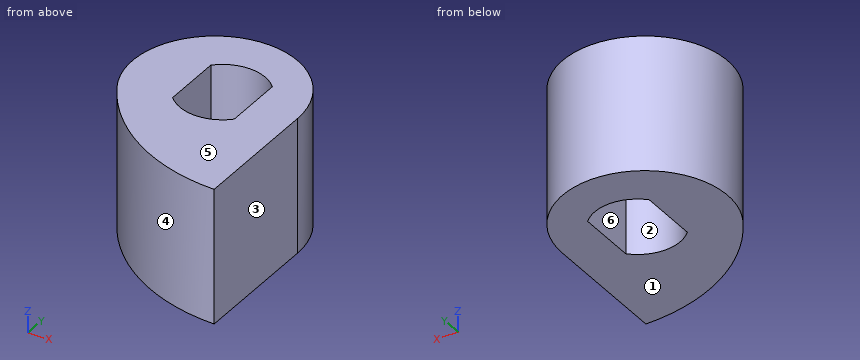
from build123d import *

# Parameters (mm, degrees)
EXTRUDE_935_DEPTH      = 4.5
EXTRUDE_935_DEPTH_BACK = 4.5


with BuildPart() as part:
    # Эскиз1 → Extrude 935 (new, two sides: drawn at the far end of the back side and taken through both)
    with BuildSketch(Plane.XY.offset(-EXTRUDE_935_DEPTH_BACK)):
        with BuildLine():
            Line((5, 0), (5, -8.660254038))
            ThreePointArc((5, -8.660254038), (-0.911767719, -7.082761379), (-5.251705953, -2.769709468))
            ThreePointArc((-5.251705953, -2.769709468), (-1.934506406, 5.309631943), (5, 0))
        make_face()
        with BuildLine():
            Line((-2.05, 1.979898987), (-2.05, -1.979898987))
            ThreePointArc((-2.05, -1.979898987), (0, -2.85), (2.05, -1.979898987))
            Line((2.05, -1.979898987), (2.05, 1.979898987))
            ThreePointArc((2.05, 1.979898987), (0, 2.85), (-2.05, 1.979898987))
        make_face(mode=Mode.SUBTRACT)
    extrude(amount=EXTRUDE_935_DEPTH + EXTRUDE_935_DEPTH_BACK)


solid = part.part
Model file for the job. Use its own axes, mm. Face numbers are marked on the shaded views. A direction names the side the tool comes from. Give positions to 0.01 mm unless a question says otherwise; leave off trailing zeros. Loops run counter-clockwise (first coordinate to the right, second up) from the corner with the lowest first, then second, coordinate; pieces in that order, holes last.
Item 1: Drop a flat-ended pin along its axis: P1, Ø2, axis at x = -4.5, z = -0.5, coming from the -Y side. Give the stop position or say it passes through.
Check values:
P1: stops at y = -5.07
Item 2: Slice it at C-C (x = -0.5). Write the cut outline in (y, z).
Check values:
outline: (-7.31, -4.5) - (-2.81, -4.5) - (-2.81, 4.5) - (-7.31, 4.5) - close; (2.81, -4.5) - (5.5, -4.5) - (5.5, 4.5) - (2.81, 4.5) - close
Item 3: Mould opens along X. For the marked faces 3, 4, 5 and 6 say: +X half, -X half, draft (parallel to the pull), parting line (faces both ways), or undercut.
Check values:
face 3: +X half
face 4: -X half
face 5: draft
face 6: undercut
Item 4: Slice it at B-B (y = 0.75). Write the cut outline in (x, z).
Check values:
outline: (-5.95, -4.5) - (-2.05, -4.5) - (-2.05, 4.5) - (-5.95, 4.5) - close; (2.05, -4.5) - (4.95, -4.5) - (4.95, 4.5) - (2.05, 4.5) - close
Item 5: Drill centre lines: line 1 along X through (y, z) = (1.5, 0.75); line 2 along Y through (x, z) = (-0.5, -3.75); line 3 along Y through (x, z) = (-1.25, -1.5). Where is each one in solid material? Low to high.
Check values:
line 1: x = -5.79 to -2.05, 2.05 to 4.79
line 2: y = -7.31 to -2.81, 2.81 to 5.5
line 3: y = -6.88 to -2.56, 2.56 to 5.45
Item 6: Which spindle directions (+Z, -Z, +X, -X, +Y, -Y) get a long thin tool onto all of the face, cutting with end or side? Do the marked faces 1 and 2. Say none if no direction does.
Check values:
face 1: -Z, +X, -X, +Y, -Y
face 2: +Z, -Z
Item 7: Slice it at A-A (z = 0.25). Write the cut outline in (x, y), plus the area to 3 significant figures.
Check values:
outline: (-5.25, -2.77) arc R11.87 ccw to (5, -8.66) - (5, 0) arc R5.5 ccw (long way) to start; hole (-2.05, -1.98) arc R2.85 ccw to (2.05, -1.98) - (2.05, 1.98) arc R2.85 ccw to (-2.05, 1.98) - close
area: 99.0 mm2
Item 8: Slice it at D-D (x = -4.5). Write the cut outline in (y, z), plus the area to 3 significant figures.
Check values:
outline: (-3.9, -4.5) - (3.77, -4.5) - (3.77, 4.5) - (-3.9, 4.5) - close
area: 69.1 mm2
